```python
from build123d import *

# Parameters (mm, degrees)
SKETCH2_R           = 15
BOSS_EXTRUDE1_DEPTH = 60
SKETCH3_R           = 5
CUT_EXTRUDE1_DEPTH  = 60
RIB1_REACH          = 102.544
SKETCH7_WALL_W      = 272.036302532
SKETCH7_WALL_H      = 10


with BuildPart() as part:
    # Sketch2 → Boss-Extrude1 (new body)
    with BuildSketch(Plane(origin=(0, 0, 0), x_dir=(1, 0, 0), z_dir=(0, 1, 0))):
        with BuildLine():
            Line((30, 0), (30, -65))
            Line((30, -65), (53, -65))
            Line((53, -65), (53, -75))
            Line((53, -75), (33, -75))
            Line((33, -75), (33, -80))
            Line((33, -80), (20, -80))
            Line((20, -80), (12, -28))
            Line((12, -28), (-12, -28))
            Line((-12, -28), (-20, -80))
            Line((-20, -80), (-33, -80))
            Line((-33, -80), (-33, -75))
            Line((-33, -75), (-53, -75))
            Line((-53, -75), (-53, -65))
            Line((-53, -65), (-30, -65))
            Line((-30, -65), (-30, 0))
            ThreePointArc((-30, 0), (0, 30), (30, 0))
        make_face()
        with Locations(Location((0, 0, 0), (0, 0, 270))):
            Circle(SKETCH2_R, mode=Mode.SUBTRACT)
    extrude(amount=-BOSS_EXTRUDE1_DEPTH)

    # Sketch3 → Cut-Extrude1 (cut)
    with BuildSketch(Plane(origin=(0, 0, 65), x_dir=(-1, 0, 0), z_dir=(0, 0, -1))):
        with Locations((-41.5, -10)):
            Circle(SKETCH3_R)
        with Locations(Location((41.5, -10, 0), (0, 0, 180))):
            Circle(SKETCH3_R)
        with Locations((41.5, -50)):
            Circle(SKETCH3_R)
        with Locations((-41.5, -50)):
            Circle(SKETCH3_R)
    extrude(amount=-CUT_EXTRUDE1_DEPTH, mode=Mode.SUBTRACT)

    # Sketch7 wall → Rib1 (add, up to next)
    with BuildSketch(Plane(origin=(41.5, -30, 32.5), x_dir=(0.333578650439, 0, 0.942722272979), z_dir=(0.942722272979, 0, -0.333578650439)), mode=Mode.PRIVATE) as rib1_sk1:
        Rectangle(SKETCH7_WALL_W, SKETCH7_WALL_H)
    rib1_tool1 = extrude(rib1_sk1.sketch, amount=-RIB1_REACH, mode=Mode.PRIVATE) - part.part
    rib1 = rib1_tool1.solids().sort_by_distance((41.5, -30, 32.5))[0]
    add(rib1)

    # Mirror1: Rib1 across plane
    add(rib1.mirror(Plane(origin=(0, 0, 0), x_dir=(0, 0, 1), z_dir=(1, 0, 0))))


solid = part.part
```
Geometry: final body of the model. Coordinates: model frame, mm. A direction names the side the tool comes from. Coordinates: 2 decimals unless noted, no trailing zeros. Order: outer loops, then holes, each group sorted by start corner. A loop starts at its lowest first (then second) coordinate and runs counter-clockwise, first axis right, second up. Notation, with made-up numbers: (69, -31) - (81, -31) arc R13 cw to (81, -25) - close; hole circle Ø2 at (72, 80.25). An arc over 180 degrees is marked (long way). Return JSON: item names as keys, results as strings. Group by question number.
1. Material intervals for line 1 along Y through (x, z) = (41.5, 69); line 2 along X through (y, z) = (-9.5, 9); line 3 along X through (y, z) = (-38, 0), sorted ascending. Write a range as [from, to].
2. Pull-direction query (X, two-part tool) for faces 1 (the face through (0, -30, 28)), 2 (the face through (-38, -25, 41)), 3 (the face through (16, -30, 54)), 4 (the face through (-41.34, -30.07, 32.05)); classes: pulls with the +X half, pulls with the -X half, needs draft (parallel to the pull), parting line crosses it, or undercut.
3. Cut plane A-A (y = -10). Output: boundary loops of the cut face in (x, z).
4. Cut plane D-D (y = -33.5). Output: boundary loops of the cut face in (x, z), plus the area to 3 significant figures.
5. Cut plane B-B (x = 41.5). Output: boundary loops of the cut face in (y, z).
6. Cut plane C-C (z = 7). Output: boundary loops of the cut face in (x, y).
7. Set-up query: faces 5 (the face through (30, -47, 32)), 6 (the face through (-43, -30, 75)), 7 (the face through (43, -30, 75)). Return all of +Z, -Z, +X, -X, +Y, -Y with unobstructed straight access to the full face (end or side cutting, diameter ignored); none if empty.
8. Pin query (flat end, axial travel): pin 1 (12 mm diameter, centred on y = -11.5, z = 58, fed in from -X); pin 2 (10 mm diameter, centred on x = 42, y = -17.5, fed in from +Z); pin 3 (10 mm diameter, centred on x = -36.5, y = -41.5, fed in from -Z); pin 4 (9 mm diameter, centred on x = -41.5, y = -10, fed in from -Z). Return the tip coordinate at first contact, or that it passes through.
Resolved:
{
 "1": {"line 1": "y = [-60, -55], [-45, -15], [-5, 0]", "line 2": "x = [-30, -12], [12, 30]", "line 3": "x = [-30, -15], [15, 30]"},
 "2": {"face 1": "undercut", "face 2": "needs draft", "face 3": "undercut", "face 4": "pulls with the -X half"},
 "3": {"outline": "(-53, 65) - (-46.5, 65) - (-46.5, 75) - (-53, 75) - close; (-36.5, 65) - (-30, 65) - (-30, 0) arc R30 ccw to (30, 0) - (30, 65) - (36.5, 65) - (36.5, 75) - (33, 75) - (33, 80) - (20, 80) - (12, 28) - (-12, 28) - (-20, 80) - (-33, 80) - (-33, 75) - (-36.5, 75) - close; (46.5, 65) - (53, 65) - (53, 75) - (46.5, 75) - close; hole circle Ø30 at (0, 0)"},
 "4": {"outline": "(-53, 65) - (-30, 0) arc R30 ccw to (30, 0) - (53, 65) - (53, 75) - (33, 75) - (33, 80) - (20, 80) - (12, 28) - (-12, 28) - (-20, 80) - (-33, 80) - (-33, 75) - (-53, 75) - close; hole circle Ø30 at (0, 0)", "area": "5,830 mm²"},
 "5": {"outline": "(-60, 65) - (-55, 65) - (-55, 75) - (-60, 75) - close; (-45, 65) - (-35, 65) - (-35, 32.5) - (-25, 32.5) - (-25, 65) - (-15, 65) - (-15, 75) - (-45, 75) - close; (-5, 65) - (0, 65) - (0, 75) - (-5, 75) - close"},
 "6": {"outline": "(-32.48, -35) - (-30, -35) - (-30, -60) - (-13.27, -60) - (-13.27, 0) - (-30, 0) - (-30, -25) - (-32.48, -25) - close; (13.27, -60) - (30, -60) - (30, -35) - (32.48, -35) - (32.48, -25) - (30, -25) - (30, 0) - (13.27, 0) - close"},
 "7": {"face 5": "-Z, +X, -Y", "face 6": "+Z, -X, +Y, -Y", "face 7": "+Z, +X, +Y, -Y"},
 "8": {"pin 1": "stops at x = -30", "pin 2": "stops at z = 75", "pin 3": "stops at z = 65", "pin 4": "passes through"}
}
